```python
from build123d import *

# Parameters (mm, degrees)
BOSS_EXTRUDE1_DEPTH = 19.05
SKETCH9_R           = 1.5875
SKETCH9_R_2         = 0.79375
CUT_EXTRUDE3_DEPTH  = 29.02437948
FILLET1_R           = 5.08


with BuildPart() as part:
    # Sketch8 → Boss-Extrude1 (new body)
    with BuildSketch(Plane(origin=(0, 0, 0), x_dir=(1, 0, 0), z_dir=(0, 1, 0))):
        with BuildLine():
            Line((-11.938, 0), (11.938, 0))
            ThreePointArc((11.938, 0), (12.539558645, -0.249173749), (12.788732394, -0.850732394))
            Line((12.788732394, -0.850732394), (12.788732394, -16.090732394))
            Line((12.788732394, -16.090732394), (11.518732394, -16.090732394))
            Line((11.518732394, -16.090732394), (11.518732394, -1.348144756))
            Line((11.518732394, -1.348144756), (-11.518727516, -1.348144756))
            Line((-11.518727516, -1.348144756), (-11.518727516, -16.090732394))
            Line((-11.518727516, -16.090732394), (-12.788727516, -16.090732394))
            Line((-12.788727516, -16.090732394), (-12.788727516, -0.850732394))
            ThreePointArc((-12.788727516, -0.850732394), (-12.539558645, -0.249173749), (-11.938, 0))
        make_face()
    extrude(amount=BOSS_EXTRUDE1_DEPTH)

    # Sketch9 → Cut-Extrude3 (cut, through all)
    with BuildSketch(Plane(origin=(0, 0, 0), x_dir=(-1, 0, 0), z_dir=(0, 0, -1))):
        with Locations((0, 9.652)):
            Circle(SKETCH9_R)
        with Locations((0, 3.302)):
            Circle(SKETCH9_R)
        with Locations((-4.7625, 16.002)):
            Circle(SKETCH9_R_2)
        with Locations((4.7625, 16.002)):
            Circle(SKETCH9_R_2)
        Polygon((-12.788732394, 16.002), (-3.224577063, 19.05), (-12.788732394, 19.05), align=None)
        Polygon((12.788732394, 16.002), (3.224577063, 19.05), (12.788729955, 19.05), align=None)
    extrude(amount=-CUT_EXTRUDE3_DEPTH, mode=Mode.SUBTRACT)

    # Fillet1
    fillet1_edges = [part.edges().sort_by_distance(p)[0] for p in [
        (3.224577063, 19.05, 0.674072378),
        (-3.224577063, 19.05, 0.674072378),
    ]]
    fillet(fillet1_edges, radius=FILLET1_R)


solid = part.part
```
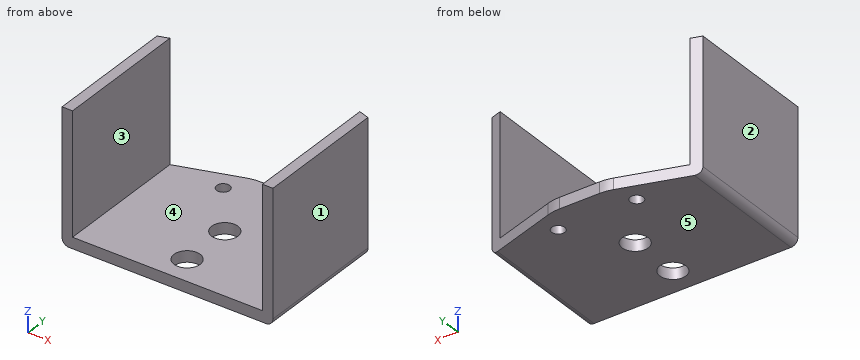
Model file for the job. Use its own axes, mm. Face numbers are marked on the shaded views. A direction names the side the tool comes from. Coordinates: 2 decimals unless noted, no trailing zeros. Write each loop counter-clockwise with the first axis right and the second up, starting at its lowest first coordinate (ties: lowest second). Pieces come first, ordered by that corner, then holes. Notation, with made-up numbers: (70.5, -32.75) - (98.5, -32.75) arc R23 ccw to (98.5, -23.75) - close; hole circle Ø6 at (76, 62.25). An arc over 180 degrees is marked (long way). One line per question, with ' | ' between items. Start each with the question number.
Q1. Cut at A-A, the plane x = 0. List the corners of the cut face in (y, z).
Q2. Drill centre lines: line 1 (Y direction, x = 0, z = 1); line 2 (X direction, y = 1, z = 11.25); line 3 (Z direction, x = 4.25, y = 14.25). Where is each one in solid material? Low to high. Write a range as [from, to].
Q3. 3-axis set-ups, long thin cutter, end or side, ignore diameter. For the marked faces 4 and 5: which of +Z, -Z, +X, -X, +Y, -Y reach the whole face in a straight line?
Q4. Pin check, flat tips, straight feed: pin 1 (3 mm diameter, centred on x = 0, y = 3.302, fed in from -Z); pin 2 (1.5 mm diameter, centred on x = 8.5, y = 6.5, fed in from +Z). Stop position of each tip, or through.
Q5. Cut at C-C, the plane y = 7.5. List the corners of the cut face in (x, z), then the cut area to 3 significant figures.
Q6. Pull direction X, two halves, no side cores. Call the marked faces 1, 2 and 3: pulls with the +X half, pulls with the -X half, needs draft (parallel to the pull), parting line crosses it, or undercut.
Q7. Cut at B-B, the plane z = 14.25. List the corners of the cut face in (x, y).
Q8. Cut at D-D, the plane x = -4.75. List the corners of the cut face in (y, z).
Answer below:
1) outline: (0, 0) - (1.71, 0) - (1.71, 1.35) - (0, 1.35) - close; (4.89, 0) - (8.06, 0) - (8.06, 1.35) - (4.89, 1.35) - close; (11.24, 0) - (19.05, 0) - (19.05, 1.35) - (11.24, 1.35) - close
2) line 1: [0, 1.71], [4.89, 8.06], [11.24, 19.05] | line 2: [-12.79, -11.52], [11.52, 12.79] | line 3: [0, 1.35]
3) face 4: +Z, +Y, -Y | face 5: -Z, +X, -X, +Y, -Y
4) pin 1: through | pin 2: z = 1.35
5) outline: (-12.79, 0.85) arc R0.85 ccw to (-11.94, 0) - (11.94, 0) arc R0.85 ccw to (12.79, 0.85) - (12.79, 16.09) - (11.52, 16.09) - (11.52, 1.35) - (-11.52, 1.35) - (-11.52, 16.09) - (-12.79, 16.09) - close | area: 71.6 mm^2
6) face 1: pulls with the +X half | face 2: pulls with the -X half | face 3: undercut
7) outline: (-12.79, 0) - (-11.52, 0) - (-11.52, 16.41) - (-12.79, 16) - close; (11.52, 0) - (12.79, 0) - (12.79, 16) - (11.52, 16.41) - close
8) outline: (0, 0) - (15.21, 0) - (15.21, 1.35) - (0, 1.35) - close; (16.8, 0) - (18.56, 0) - (18.56, 1.35) - (16.8, 1.35) - close
